Can you work these out from the model? Positions are in its coordinate system, mm. A direction names the side the tool comes from. Coordinates: 2 decimals unless noted, no trailing zeros. Order: outer loops, then holes, each group sorted by start corner. A loop starts at its lowest first (then second) coordinate and runs counter-clockwise, first axis right, second up. Notation, with made-up numbers: (-1, 72) -> (57, 72) arc R19 cw to (57, 81) -> close; hole circle Ø5 at (82, 39.25). An arc over 180 degrees is marked (long way). Write item = value, one per line.
Autodesk Inventor part; units mm, degrees
ref_plane "YZ Plane" through (0, 0, 0) normal (1, 0, 0) x (0, 1, 0)
ref_plane "XZ Plane" through (0, 0, 0) normal (0, 1, 0) x (-1, 0, 0)
ref_plane "XY Plane" through (0, 0, 0) normal (0, 0, 1) x (1, 0, 0)
sketch "Sketch1" plane through (0, 0, 0) normal (0, 1, 0) x (-1, 0, 0)
  line L0 (0, -28.84) -> (0, 33.04)
  line L1 (39.2, 0) -> (-39.2, 0)
  line L2 (-28, 10) -> (-28, -10)
  line L3 (28, 10) -> (28, -10)
  line L4 (-28, 10) -> (-2.6, 10)
  line L5 (-2.6, 10) -> (-2.6, 0)
  line L6 (28, 10) -> (2.6, 10)
  line L7 (2.6, 10) -> (2.6, 0)
  arc A0 (-2.6, 0) -> (2.6, 0) centre (0, 0) ccw
  arc A1 (-28, -10) -> (28, -10) centre (0, 24.2) ccw
  dimension "d0" = 5.2
  dimension "d1" = 56
  dimension "d2" = 20
  dimension "d3" = 10
  dimension "d4" = 20
extrude "Extrusion1" add sketch "Sketch1" along normal blind 8 contours A1 L2 L1 A0 L0 | L0 A0 L1 L3 A1 | L1 L2 L4 L5 | L7 L6 L3 L1
sketch "Sketch2" plane through (0, 0, 0) normal (0, 0, 1) x (1, 0, 0)
  arc A0 (5.1, 0) -> (0, 5.1) centre (0, 0) ccw
  line L0 (0, -1.2312) -> (0, 7.3875)
  line L1 (0, 5.1) -> (0, 0)
  line L2 (0, 0) -> (5.1, 0)
  dimension "d7" = 10.2
revolve "Revolution1" cut sketch "Sketch2" angle 360 about axis through (0, -10, 0) along (0, 1, 0)
sketch "Sketch4" plane through (0, 8, 0) normal (0, 1, 0) x (1, 0, 0)
  line L0 (0, 26) -> (0, -16)
  line L1 (28, -10) -> (28, 10)
  line L2 (39.2, 0) -> (-39.2, 0)
  point P0 (0, 0)
  point P1 (18, 0)
  point P2 (-18, 0)
  dimension "d9" = 10
hole "Hole1" at (18, 8, 0) at (-18, 8, 0) direction (0, -1, 0) diameter 4.2 end through all counterbore diameter 8.65 counterbore depth 3.1
fillet "Fillet1" radius 2 6 edges at (28, 4, 10) (28, 4, -10) (-28, 4, -10) (-28, 4, 10) (-2.6, 4, 10) (2.6, 4, 10)
sketch "Sketch5" plane through (0, 0, 0) normal (0, 0, 1) x (1, 0, 0)
  line L0 (4.6, 0) -> (26, 0)
  arc A0 (5.1, 0) -> (-5.1, 0) centre (0, 0) ccw
  line L1 (5.1, 0) -> (-5.1, 0)
  line L2 (-5.1, 0) -> (5.1, 0)
  point P0 (2.6, 0)
  point P1 (-2.6, 0)
  dimension "d18" = 5.1
extrude "Extrusion2" cut sketch "Sketch5" along normal blind 10
properties part number "Kameralefogov3"
Item 1: I want a section at D-D, the plane z = -11.5. Please give me the cut outline in (x, y).
A:
outline = (-26.06, 0) -> (26.06, 0) -> (26.06, 8) -> (-26.06, 8) -> close
Item 2: I want a section at B-B, the plane x = 18. Please give me the cut outline in (y, z) (3 decimals), plus the area to 3 significant figures.
A:
outline = (0, -16.169) -> (8, -16.169) -> (8, -4.325) -> (4.9, -4.325) -> (4.9, -2.1) -> (0, -2.1) -> close; (0, 2.1) -> (4.9, 2.1) -> (4.9, 4.325) -> (8, 4.325) -> (8, 10) -> (0, 10) -> close
area = 162 mm2
Item 3: I want a section at C-C, the plane x = 0. Please give me the cut outline in (y, z).
A:
outline = (0, -20) -> (8, -20) -> (8, -2.6) -> (4.39, -2.6) arc R5.1 cw to (0, -5.1) -> close
Item 4: If we mould it in two halves opening along X, with no side actions, what happens to faces 4 (the cylindrical face through (0, 4, -20)), 5 (the flat face through (-15, 4, 10)), 6 (the cylindrical face through (-22.29, 6.43, -0.56)), 7 (the flat face through (28, 4, 0))? For each: pulls with the +X half, pulls with the -X half, needs draft (parallel to the pull), parting line crosses it, or undercut.
A:
face_4 = parting line crosses it
face_5 = needs draft
face_6 = undercut
face_7 = pulls with the +X half
Item 5: For faces 1 (the cylindrical face through (13.71, 6.43, -0.56)), 2 (the cylindrical face through (-4.45, 2.49, 4.93)), 3 (the flat face through (2.6, 6, 4)), which set-ups out of +Z, -Z, +X, -X, +Y, -Y let a thin tool reach every point of the face, with its end or its side?
A:
face_1 = +Y
face_2 = +Z, -Y
face_3 = +Z, +Y, -Y
Item 6: If I drill on probe 1 along X at (y, z) = (6.85, 0) (3 decimals); probe 2 along X at (y, z) = (3, 0); probe 3 along X at (y, z) = (5.25, -3.5), over which ranges is the centre line in solid material (lowest first)?
A:
probe_1 = -28 to -22.325, -13.675 to -2.6, 2.6 to 13.675, 22.325 to 28
probe_2 = -28 to -20.1, -15.9 to -4.12, 4.12 to 15.9, 20.1 to 28
probe_3 = -28 to -20.54, -15.46 to 15.46, 20.54 to 28
Item 7: I want a section at A-A, the plane y = 1. Please give me the cut outline in (x, z).
A:
outline = (-28, -9.04) arc R2 ccw to (-27.23, -10.61) arc R44.2 ccw to (27.23, -10.61) arc R2 ccw to (28, -9.04) -> (28, 8) arc R2 ccw to (26, 10) -> (5, 10) -> (5, 0) arc R5 cw to (-5, 0) -> (-5, 10) -> (-26, 10) arc R2 ccw to (-28, 8) -> close; hole circle Ø4.2 at (-18, 0); hole circle Ø4.2 at (18, 0)
Item 8: I'm going to push flat-ended pins straight in: P1, Ø4.5, axis at x = -18, z = -0.5, coming from the +Y side; P2, Ø4, axis at x = -16, y = 3.5, coming from the -Z side; P3, Ø3.5, axis at x = 18, z = 0, coming from the -Y side; P4, Ø3, axis at x = 4.5, y = 2.5, coming from the -Z side. Where does each tip first touch, or does it pass through?
A:
P1 = 4.9
P2 = -17.72
P3 = through
P4 = -19.9
